Autodesk Inventor part; units mm, degrees
ref_plane "YZ Plane" through (0, 0, 0) normal (1, 0, 0) x (0, 1, 0)
ref_plane "XZ Plane" through (0, 0, 0) normal (0, 1, 0) x (-1, 0, 0)
ref_plane "XY Plane" through (0, 0, 0) normal (0, 0, 1) x (1, 0, 0)
sketch "スケッチ1" plane through (0, 0, 0) normal (1, 0, 0) x (0, 1, 0)
  line L0 (-167.5617, 195.4399) -> (192.4383, 195.4399)
  line L1 (192.4383, 195.4399) -> (192.4383, 180.4399)
  line L2 (192.4383, 180.4399) -> (-167.5617, 180.4399)
  line L3 (-167.5617, 180.4399) -> (-167.5617, 195.4399)
  line L4 (-167.5617, 230.4399) -> (-182.5617, 230.4399)
  line L5 (-182.5617, 230.4399) -> (-182.5617, 2.9399)
  line L6 (-182.5617, 2.9399) -> (-167.5617, 2.9399)
  line L7 (-167.5617, 2.9399) -> (-167.5617, 230.4399)
  line L8 (-167.5617, 230.4399) -> (-182.5617, 230.4399)
  line L9 (-182.5617, 230.4399) -> (-182.5617, 215.4399)
  line L10 (-182.5617, 215.4399) -> (-167.5617, 215.4399)
  line L11 (-167.5617, 215.4399) -> (-167.5617, 230.4399)
  line L12 (-117.5617, 180.4399) -> (-102.5617, 180.4399)
  line L13 (-102.5617, 180.4399) -> (-102.5617, 2.9399)
  line L14 (-102.5617, 2.9399) -> (-117.5617, 2.9399)
  line L15 (-117.5617, 2.9399) -> (-117.5617, 180.4399)
  line L16 (192.4383, 180.4399) -> (177.4383, 180.4399)
  line L17 (177.4383, 180.4399) -> (177.4383, 2.9399)
  line L18 (177.4383, 2.9399) -> (192.4383, 2.9399)
  line L19 (192.4383, 2.9399) -> (192.4383, 180.4399)
  circle A0 centre (-142.5617, 135.4399) radius 12.5
  circle A1 centre (-142.5617, 95.4399) radius 18.75
  line L20 (192.4383, 2.9399) -> (-167.5617, 2.9399)
  line L21 (-182.5617, 155.4399) -> (-102.5617, 155.4399)
  line L22 (-102.5617, 75.4399) -> (-182.5617, 75.4399)
  circle A2 centre (-142.5617, 95.4399) radius 20
  line L23 (-125.0617, 195.4399) -> (-125.0617, 180.4399)
  line L24 (-102.5617, 180.4399) -> (-102.5617, 195.4399)
  line L25 (-147.5617, 195.4399) -> (-147.5617, 180.4399)
  line L26 (-167.5617, 202.9399) -> (-182.5617, 202.9399)
  line L27 (-167.5617, 172.9399) -> (-182.5617, 172.9399)
  circle A3 centre (157.4383, 135.4399) radius 12.5
  line L28 (192.4383, 160.4399) -> (177.4383, 160.4399)
  line L29 (169.9383, 195.4399) -> (169.9383, 180.4399)
  line L30 (-167.5617, -189.5601) -> (192.4383, -189.5601)
  line L31 (192.4383, -189.5601) -> (192.4383, -174.5601)
  line L32 (192.4383, -174.5601) -> (-167.5617, -174.5601)
  line L33 (-167.5617, -174.5601) -> (-167.5617, -189.5601)
  line L34 (-167.5617, -224.5601) -> (-182.5617, -224.5601)
  line L35 (-182.5617, -224.5601) -> (-182.5617, 2.9399)
  line L36 (-167.5617, 2.9399) -> (-167.5617, -224.5601)
  line L37 (-167.5617, -224.5601) -> (-182.5617, -224.5601)
  line L38 (-182.5617, -224.5601) -> (-182.5617, -209.5601)
  line L39 (-182.5617, -209.5601) -> (-167.5617, -209.5601)
  line L40 (-167.5617, -209.5601) -> (-167.5617, -224.5601)
  line L41 (-117.5617, -174.5601) -> (-102.5617, -174.5601)
  line L42 (-102.5617, -174.5601) -> (-102.5617, 2.9399)
  line L43 (-117.5617, 2.9399) -> (-117.5617, -174.5601)
  line L44 (192.4383, -174.5601) -> (177.4383, -174.5601)
  line L45 (177.4383, -174.5601) -> (177.4383, 2.9399)
  line L46 (192.4383, 2.9399) -> (192.4383, -174.5601)
  circle A4 centre (-142.5617, -129.5601) radius 12.5
  circle A5 centre (-142.5617, -89.5601) radius 18.75
  line L47 (-182.5617, -149.5601) -> (-102.5617, -149.5601)
  line L48 (-102.5617, -69.5601) -> (-182.5617, -69.5601)
  circle A6 centre (-142.5617, -89.5601) radius 20
  line L49 (-125.0617, -189.5601) -> (-125.0617, -174.5601)
  line L50 (-102.5617, -174.5601) -> (-102.5617, -189.5601)
  line L51 (-147.5617, -189.5601) -> (-147.5617, -174.5601)
  line L52 (-167.5617, -197.0601) -> (-182.5617, -197.0601)
  line L53 (-167.5617, -167.0601) -> (-182.5617, -167.0601)
  circle A7 centre (157.4383, -129.5601) radius 12.5
  line L54 (192.4383, -154.5601) -> (177.4383, -154.5601)
  line L55 (169.9383, -189.5601) -> (169.9383, -174.5601)
  line L56 (192.4383, 155.4399) -> (144.9383, 155.4399)
  line L57 (144.9383, 155.4399) -> (144.9383, 75.4399)
  line L58 (144.9383, 75.4399) -> (192.4383, 75.4399)
  line L59 (192.4383, 75.4399) -> (192.4383, 155.4399)
  line L60 (177.4383, 155.4399) -> (153.4158, 147.275)
  line L61 (146.595, 129.2213) -> (177.4383, 75.4399)
  circle A8 centre (-175.0617, 197.9399) radius 1.7
  circle A9 centre (-175.0617, 187.9399) radius 1.7
  circle A10 centre (-175.0617, 177.9399) radius 1.7
  circle A11 centre (-162.5617, 187.9399) radius 1.7
  circle A12 centre (-152.5617, 187.9399) radius 1.7
  point P0 (0, 0)
  point P1 (-120.0617, 187.9399)
  point P2 (-110.0617, 187.9399)
  point P3 (-110.0617, 175.4399)
  point P4 (-110.0617, 165.4399)
  point P5 (184.9383, 175.4399)
  point P6 (184.9383, 165.4399)
  point P7 (184.9383, 187.9399)
  point P8 (174.9383, 187.9399)
  point P9 (-110.0617, 180.4399)
  point P10 (192.4383, 187.9399)
  point P11 (-110.0617, 95.4399)
  point P12 (-110.0617, 135.4399)
  point P13 (-175.0617, 135.4399)
  point P14 (-175.0617, 95.4399)
  point P15 (-175.0617, -89.5601)
  point P16 (-110.0617, -89.5601)
  point P17 (-110.0617, -129.5601)
  point P18 (-175.0617, -129.5601)
  point P19 (-175.0617, -172.0601)
  point P20 (-175.0617, -182.0601)
  point P21 (-175.0617, -192.0601)
  point P22 (-162.5617, -182.0601)
  point P23 (-152.5617, -182.0601)
  point P24 (-120.0617, -182.0601)
  point P25 (-110.0617, -182.0601)
  point P26 (-110.0617, -169.5601)
  point P27 (-110.0617, -159.5601)
  point P28 (174.9383, -182.0601)
  point P29 (184.9383, -182.0601)
  point P30 (184.9383, -169.5601)
  point P31 (184.9383, -159.5601)
  point P32 (184.9383, 135.4399)
  point P33 (184.9383, 95.4399)
  point P34 (177.4383, 91.6899)
  point P35 (184.9383, -89.5601)
  point P36 (184.9383, -129.5601)
  dimension "d0" = 7.5
  dimension "d1" = 7.5
  dimension "d2" = 7.5
  dimension "d3" = 7.5
  dimension "d4" = 10
  dimension "d5" = 10
  dimension "d6" = 5
  dimension "d7" = 10
  dimension "d8" = 7.5
  dimension "d9" = 7.5
  dimension "d10" = 7.5
  dimension "d11" = 10
  dimension "d12" = 7.5
  dimension "d13" = 7.5
  dimension "d14" = 5
  dimension "d15" = 10
  dimension "d16" = 7.5
  dimension "d17" = 7.5
  dimension "d18" = 7.5
  dimension "d19" = 10
  dimension "d20" = 7.5
  dimension "d21" = 7.5
  dimension "d22" = 5
  dimension "d23" = 10
  dimension "d24" = 7.5
  dimension "d25" = 7.5
  dimension "d26" = 20
  dimension "d27" = 20
  dimension "d28" = 7.5
  dimension "d29" = 7.5
  dimension "d30" = 20
  dimension "d31" = 7.5
  dimension "d32" = 7.5
  dimension "d33" = 20
  dimension "d34" = 3.4
  dimension "d35" = 3.4
  dimension "d36" = 3.4
  dimension "d37" = 3.4
  dimension "d38" = 3.4
extrude "押し出し1" add sketch "スケッチ1" along normal blind 5 contours L0 L25 L2 L3 | L3 L7 L27 L5 L26
fillet "フィレット1" radius 2 8 edges at (2.5, -147.5617, 195.4399) (2.5, -167.5617, 195.4399) (2.5, -167.5617, 202.9399) (2.5, -182.5617, 202.9399) (2.5, -182.5617, 172.9399) (2.5, -167.5617, 172.9399) (2.5, -167.5617, 180.4399) (2.5, -147.5617, 180.4399)
properties part number "ball_loading_v1_Plate_ASP_F_1" material "ABS プラスチック"
Geometry check sheet. Reference: the model listing, model coordinates, mm. A direction names the side the tool comes from. Give positions to 0.01 mm unless a question says otherwise; leave off trailing zeros. Order: outer loops, then holes, each group sorted by start corner. A loop starts at its lowest first (then second) coordinate and runs counter-clockwise, first axis right, second up. Notation, with made-up numbers: (-33.75, -31.5) -> (-7.75, -31.5) arc R11 cw to (-7.75, -12.5) -> close; hole circle Ø6 at (72.25, 84). An arc over 180 degrees is marked (long way). Write each question's results on one line, items separated by ' | '. Start each with the question number.
(1) Gauge pin test, flat ends, axial feed: P1, Ø1.8, axis at x = 2.5, z = 177.5, coming from the +Y side; P2, Ø2.5, axis at x = 3.5, y = -161, coming from the +Z side; P3, Ø2, axis at y = -162.56, z = 187.94, coming from the -X side; P4, Ø3, axis at x = 0.5, z = 198, coming from the +Y side. Record the tip position at first contact, or that the pin passes through.
(2) Scan lines: line 1 (Z direction, x = 2.3, y = -175); line 2 (Y direction, x = 1.5, z = 188); line 3 (Z direction, x = 3.95, y = -162.5). Record each from-to range of solid material in increasing order.
(3) Sectioned sample at C-C (x = 3.1). Enter the section's corners in (y, z).
(4) Sectioned sample at D-D (y = -152). Enter the section's corners in (x, z).
(5) Sectioned sample at A-A (z = 189). Enter the section's corners in (x, y), plus the area to 3 significant figures.
(6) Access from +Z, -Z, +X, -X, +Y, -Y to the whole of each face (thin tool, end or side, straight path). Record for faces 1 (the face through (2, -167.562, 199)), 2 (the face through (2, -167.562, 177)), 3 (the face through (2.465, -151.648, 186.506)).
(7) Sectioned sample at B-B (y = -175.5). Enter the section's corners in (x, z).
(8) Mould release check, pull along Y, two halves, no side actions. Record for faces 4 (the face through (2.465, -161.648, 186.506)), 5 (the face through (2, -157, 180.44)), 6 (the face through (2.535, -168.132, 202.338)): pulls with the +Y half, pulls with the -Y half, needs draft (parallel to the pull), parting line crosses it, or undercut.
Answer below:
1) P1: y = -167.56 | P2: z = 195.44 | P3: through | P4: y = -167.33
2) line 1: 172.94 to 176.24, 179.64 to 186.24, 189.64 to 196.24, 199.64 to 202.94 | line 2: -182.56 to -176.76, -173.36 to -164.26, -160.86 to -154.26, -150.86 to -147.56 | line 3: 180.44 to 186.24, 189.64 to 195.44
3) outline: (-182.56, 174.94) arc R2 ccw to (-180.56, 172.94) -> (-169.56, 172.94) arc R2 ccw to (-167.56, 174.94) -> (-167.56, 178.44) arc R2 cw to (-165.56, 180.44) -> (-149.56, 180.44) arc R2 ccw to (-147.56, 182.44) -> (-147.56, 193.44) arc R2 ccw to (-149.56, 195.44) -> (-165.56, 195.44) arc R2 cw to (-167.56, 197.44) -> (-167.56, 200.94) arc R2 ccw to (-169.56, 202.94) -> (-180.56, 202.94) arc R2 ccw to (-182.56, 200.94) -> close; hole circle Ø3.4 at (-175.06, 177.94); hole circle Ø3.4 at (-175.06, 187.94); hole circle Ø3.4 at (-175.06, 197.94); hole circle Ø3.4 at (-162.56, 187.94); hole circle Ø3.4 at (-152.56, 187.94)
4) outline: (0, 180.44) -> (5, 180.44) -> (5, 186.34) -> (0, 186.34) -> close; (0, 189.54) -> (5, 189.54) -> (5, 195.44) -> (0, 195.44) -> close
5) outline: (0, -182.56) -> (5, -182.56) -> (5, -176.39) -> (0, -176.39) -> close; (0, -173.73) -> (5, -173.73) -> (5, -163.89) -> (0, -163.89) -> close; (0, -161.23) -> (5, -161.23) -> (5, -153.89) -> (0, -153.89) -> close; (0, -151.23) -> (5, -151.23) -> (5, -147.56) -> (0, -147.56) -> close | area: 135 mm2
6) face 1: +Z, +X, -X, +Y | face 2: -Z, +X, -X, +Y | face 3: +X, -X
7) outline: (0, 172.94) -> (5, 172.94) -> (5, 176.3) -> (0, 176.3) -> close; (0, 179.58) -> (5, 179.58) -> (5, 186.3) -> (0, 186.3) -> close; (0, 189.58) -> (5, 189.58) -> (5, 196.3) -> (0, 196.3) -> close; (0, 199.58) -> (5, 199.58) -> (5, 202.94) -> (0, 202.94) -> close
8) face 4: undercut | face 5: needs draft | face 6: pulls with the +Y half
